Could you check a few things on this model? Use its own coordinates, in mm. Round coordinates to 2 decimals unless told otherwise and drop trailing zeros. Loops run counter-clockwise (first coordinate to the right, second up) from the corner with the lowest first, then second, coordinate; pieces in that order, holes last. Notation, with made-up numbers: M 25.5,-15.75 L 84.5,-15.75 A28 ccw 84.5,12.25 Z; hole C 73.25,30 d5. An arc over 180 degrees is marked long. Answer in a Markdown table with one row per item.
```python
from build123d import *

# Parameters (mm, degrees)
BASPROSKE_W        = 3.175
BASPROSKE_H        = 6.35
TOOTHCUT_DEPTH     = 10.525
TEETHCUTS_COUNT    = 10
TEETHCUTS_ANGLE    = 324
BORSKE_R           = 0.99949
BORE_DEPTH         = 50.8000508
CUT_EXTRUDE1_DEPTH = 10.344170464


with BuildPart() as part:
    # BasProSke → Base-Revolve (revolve)
    with BuildSketch(Plane(origin=(0, 0, 0), x_dir=(1, 0, 0), z_dir=(0, 1, 0)), mode=Mode.PRIVATE) as base_revolve_sk:
        with Locations((1.5875, 3.175)):
            Rectangle(BASPROSKE_W, BASPROSKE_H)
    revolve(base_revolve_sk.sketch.rotate(Axis((-10, 0, 0), (1, 0, 0)), 180), axis=Axis((-10, 0, 0), (1, 0, 0)))

    # TooCutSke → ToothCut (cut, through all)
    with BuildSketch(Plane(origin=(0, 0, 0), x_dir=(0, 0, -1), z_dir=(1, 0, 0))):
        with BuildLine():
            ThreePointArc((0.630210727, 3.920537785), (0, 3.970866667), (-0.630210727, 3.920537785))
            ThreePointArc((-0.630210727, 3.920537785), (-0.900510691, 5.2110639), (-1.88228345, 6.091201374))
            ThreePointArc((-1.88228345, 6.091201374), (0, 6.3754), (1.88228345, 6.091201374))
            ThreePointArc((1.88228345, 6.091201374), (0.900510691, 5.2110639), (0.630210727, 3.920537785))
        make_face()
    toothcut = extrude(amount=TOOTHCUT_DEPTH, mode=Mode.SUBTRACT)

    # TeethCuts: ToothCut ×10 about axis
    teethcuts_axis = Axis((-10, 0, 0), (1, 0, 0))
    for i in range(1, TEETHCUTS_COUNT):
        add(toothcut.rotate(teethcuts_axis, i * TEETHCUTS_ANGLE / (TEETHCUTS_COUNT - 1)), mode=Mode.SUBTRACT)

    # BorSke → Bore (cut, symmetric)
    with BuildSketch(Plane(origin=(0, 0, 0), x_dir=(0, 0, -1), z_dir=(1, 0, 0))):
        with Locations(Location((0, 0, 0), (0, 0, 180))):
            Circle(BORSKE_R)
    extrude(amount=BORE_DEPTH, both=True, mode=Mode.SUBTRACT)

    # Sketch1 → Cut-Extrude1 (cut, through all)
    with BuildSketch(Plane(origin=(3.175, 0, 0), x_dir=(0, 0, -1), z_dir=(1, 0, 0))):
        with BuildLine():
            Line((-1.207769332, 1.27), (1.207769332, 1.27))
            ThreePointArc((1.207769332, 1.27), (0, -1.7526), (-1.207769332, 1.27))
        make_face()
    extrude(amount=-CUT_EXTRUDE1_DEPTH, mode=Mode.SUBTRACT)


solid = part.part
```
1) If we mould it in two halves opening along Z, with no side actions, what happens to faces 1 (the face through (0, 1, 2)), 2 (the face through (1.57, 3.67, 3.76))? For each: released by +Z, released by -Z, zero draft, split by the parting line, or undercut.
Computed:
| item | result |
|---|---|
| face 1 | zero draft |
| face 2 | undercut |
2) I want a section at B-B, the plane y = 4.5. Please give me the cut outline in (x, z) (3 decimals), plus the area to 3 significant figures.
Computed:
| item | result |
|---|---|
| outline | M 0,-2.294 L 3.175,-2.294 L 3.175,-0.646 L 0,-0.646 Z; M 0,0.646 L 3.175,0.646 L 3.175,2.294 L 0,2.294 Z |
| area | 10.5 mm² |
3) I want a section at A-A, the plane z = 0. Please give me the cut outline in (x, y) (3 decimals), plus the area to 3 significant figures.
Computed:
| item | result |
|---|---|
| outline | M 0,-3.971 L 3.175,-3.971 L 3.175,-1.753 L 0,-1.753 Z; M 0,1.27 L 3.175,1.27 L 3.175,3.971 L 0,3.971 Z |
| area | 15.6 mm² |
4) Will these pins go through, and if not, where does the flat tip stop? P1, Ø1.5, axis at x = 1, y = -3.5, coming from the -Z side; P2, Ø1.5, axis at x = 2, z = -1, coming from the -Y side; P3, Ø3, axis at y = 0, z = 0, coming from the +X side (3 decimals); P4, Ø0.7, axis at x = 2, z = -0.5, coming from the -Y side.
Computed:
| item | result |
|---|---|
| P1 | stops at z = -5.21 |
| P2 | stops at y = -6.03 |
| P3 | stops at x = 3.175 |
| P4 | stops at y = -5.12 |
5) I need wall thicknesses on line 1 (Z direction, x = 1.2, y = 0); line 2 (Y direction, x = 3, z = 5); line 3 (Z direction, x = 1.5, y = -3.5). Which ranges of each line are inside material? Lowest first, please.
Computed:
| item | result |
|---|---|
| line 1 | z = -6.35 to -1.75, 1.75 to 6.35 |
| line 2 | y = -3.84 to -2.94, -0.79 to 0.79, 2.94 to 3.84 |
| line 3 | z = -5.19 to -3.46, -1.88 to 1.88, 3.46 to 5.19 |
6) I want a section at C-C, the plane z = 4.5. Please give me the cut outline in (x, y) (3 decimals).
Computed:
| item | result |
|---|---|
| outline | M 0,-3.864 L 3.175,-3.864 L 3.175,-2.291 L 0,-2.291 Z; M 0,-0.779 L 3.175,-0.779 L 3.175,0.779 L 0,0.779 Z; M 0,2.291 L 3.175,2.291 L 3.175,3.864 L 0,3.864 Z |
